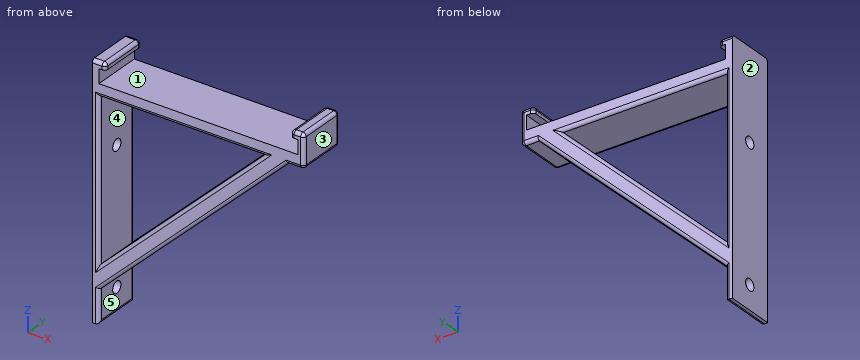
from build123d import *

# Parameters (mm, degrees)
F1_DEPTH      = 30
F2_R          = 3.5
F3_DEPTH      = 73.1
F4_DEPTH      = 25
F4_DEPTH_BACK = 25
F5_R          = 2


with BuildPart() as f1:
    # F0 (on Front) → F1 (new body)
    with BuildSketch(Plane.XZ):
        Polygon((-57.971305, 24.073915), (-57.971305, 32.573915), (-53.971305, 32.573915), (-53.971305, 36.573915), (-61.971305, 36.573915), (-61.971305, -113.426085), (-57.971305, -113.426085), (-57.971305, -93.426085), (56.528695, 16.573915), (66.528695, 16.573915), (66.528695, 36.573915), (58.528695, 36.573915), (58.528695, 32.573915), (63.028695, 32.573915), (63.028695, 24.073915), align=None)
        Polygon((-57.971305, -79.559067), (-57.971305, 16.573915), (42.094389, 16.573915), align=None, mode=Mode.SUBTRACT)
    extrude(amount=F1_DEPTH)

    # F2 (on Right) → F3 (cut)
    with BuildSketch(Plane.YZ):
        with Locations((-14.8, -98.926085)):
            Circle(F2_R)
        with Locations((-14.8, -17.926085)):
            Circle(F2_R)
    extrude(amount=-F3_DEPTH, mode=Mode.SUBTRACT)

    # F2 (on Right) → F4 (cut, two sides)
    with BuildSketch(Plane.YZ) as f4_sk:
        with Locations((-14.8, -98.926085)):
            Circle(F2_R)
        with Locations((-14.8, -17.926085)):
            Circle(F2_R)
    extrude(amount=F4_DEPTH, mode=Mode.SUBTRACT)
    extrude(f4_sk.sketch, amount=-F4_DEPTH_BACK, mode=Mode.SUBTRACT)

    # F5
    f5_edges = [f1.edges().sort_by_distance(p)[0] for p in [
        (66.528695, -15, 36.573915),
        (58.528695, -15, 36.573915),
        (66.528695, -30, 26.573915),
        (62.528695, -30, 36.573915),
        (62.528695, 0, 36.573915),
        (66.528695, 0, 26.573915),
        (58.528695, 0, 34.573915),
        (58.528695, -30, 34.573915),
        (66.528695, -15, 16.573915),
        (61.528695, -30, 16.573915),
        (61.528695, 0, 16.573915),
        (-7.938458, -30, 16.573915),
        (-7.938458, 0, 16.573915),
        (-0.721305, -30, -38.426085),
        (-7.938458, -30, -31.492576),
        (-57.971305, -30, -31.492576),
        (-57.971305, 0, -31.492576),
        (-0.721305, 0, -38.426085),
        (-7.938458, 0, -31.492576),
        (-57.971305, -15, -113.426085),
        (-57.971305, 0, -103.426085),
        (-57.971305, -30, -103.426085),
        (-57.971305, 0, 36.573915),
        (-53.971305, 0, 34.573915),
        (-53.971305, -15, 36.573915),
        (-57.971305, -30, 36.573915),
        (-53.971305, -30, 34.573915),
    ]]
    fillet(f5_edges, radius=F5_R)


solid = f1.part
Input: part model. Units: mm. Frame: model coordinates. Face numbers are marked on the shaded views. A direction names the side the tool comes from. Give positions to 0.01 mm unless a question says otherwise; leave off trailing zeros. Order: outer loops, then holes, each group sorted by start corner. A loop starts at its lowest first (then second) coordinate and runs counter-clockwise, first axis right, second up.
Q1. Contact query for flat-ended pins moving along their axis: pin 1 Ø8 at (y, z) = (-14.8, -17.93) entering from -X; pin 2 Ø10 at (y, z) = (-4.5, -70) entering from +X; pin 3 Ø8 at (x, y) = (-5.5, -20.5) entering from -Z; pin 4 Ø3.5 at (x, y) = (60.5, -9.5) entering from -Z. Output: stop coordinate, or through.
Checked values:
pin 1: stops at x = -61.97
pin 2: stops at x = -28.38
pin 3: stops at z = -46.86
pin 4: stops at z = 16.57
Q2. Draft query along X for the marked faces 1, 2 and 3. Return one class per face: +X half, -X half, draft (parallel to the pull), parting line (faces both ways), or undercut.
Checked values:
face 1: undercut
face 2: -X half
face 3: +X half
Q3. Section B-B on x = 14. State how many separate pieces and enclosed holes the cut face has, and give its area (3 significant figures).
Checked values:
separate pieces: 2
enclosed holes: 1
area: 596 mm2
Q4. Ray query, probe 1 along Z at (x, y) = (-59.9, -14.8); probe 2 along Z at (x, y) = (-59, -14); probe 3 along X at (y, z) = (-18.5, -8). Return the intervals inside material, ascending.
Checked values:
probe 1: z = -113.42 to -102.43, -95.43 to -21.43, -14.43 to 36.57
probe 2: z = -113.17 to -102.33, -95.52 to -21.33, -14.52 to 36.57
probe 3: x = -61.97 to -57.97, 16.52 to 30.95
Q5. Set-up query: the marked faces 4 and 5. Return all of +Z, -Z, +X, -X, +Y, -Y with unobstructed straight access to the full face (end or side cutting, diameter ignored); none if empty.
Checked values:
face 4: +Y, -Y
face 5: -Z, +X, +Y, -Y
Q6. Section A-A on y = -9.5. Output: boundary loops of the cut face in (x, z), and give its area (3 significant figures).
Checked values:
outline: (-61.97, -113.43) - (-59.97, -113.43) arc R2 ccw to (-57.97, -111.43) - (-57.97, -93.43) - (56.53, 16.57) - (64.53, 16.57) arc R2 ccw to (66.53, 18.57) - (66.53, 34.57) arc R2 ccw to (64.53, 36.57) - (60.53, 36.57) arc R2 ccw to (58.53, 34.57) - (58.53, 32.57) - (63.03, 32.57) - (63.03, 24.07) - (-57.97, 24.07) - (-57.97, 32.57) - (-53.97, 32.57) - (-53.97, 34.57) arc R2 ccw to (-55.97, 36.57) - (-61.97, 36.57) - close; hole (-57.97, -79.56) - (42.09, 16.57) - (-57.97, 16.57) - close
area: 3,090 mm2
